For this review, take the finished solid that the model builds, in its own axes (mm). Face numbers are marked on the shaded views. A direction names the side the tool comes from. Round coordinates to 2 decimals unless told otherwise and drop trailing zeros. Write each loop counter-clockwise with the first axis right and the second up, starting at its lowest first coordinate (ties: lowest second). Pieces come first, ordered by that corner, then holes. Notation, with made-up numbers: (35, 7) -> (81, 7) arc R19 ccw to (81, 22) -> close; hole circle Ø11 at (23.5, 53.25). An arc over 180 degrees is marked (long way). Answer in a Markdown table with one row per item.
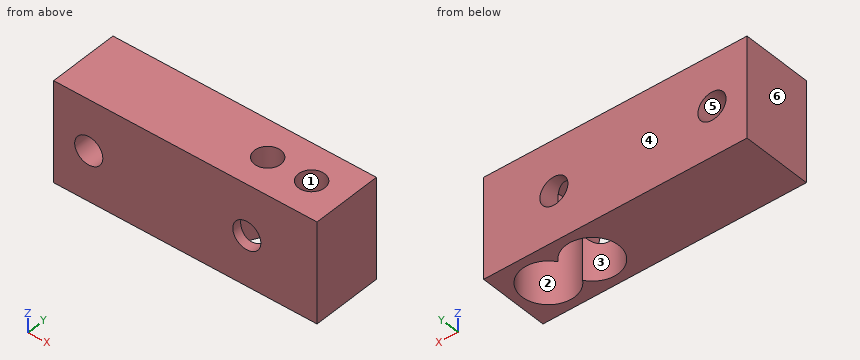
from build123d import *

# Parameters (mm, degrees)
SKETCH1_W           = 30
SKETCH1_H           = 11.5
BOSS_EXTRUDE1_DEPTH = 8
SKETCH2_R           = 1.5
CUT_EXTRUDE1_DEPTH  = 12.5
SKETCH3_R           = 1.598160281
SKETCH3_R_2         = 1.600993429
CUT_EXTRUDE2_DEPTH  = 10
CUT_EXTRUDE3_DEPTH  = 9


with BuildPart() as part:
    # Sketch1 → Boss-Extrude1 (new body)
    with BuildSketch(Plane(origin=(0, 0, 0), x_dir=(1, 0, 0), z_dir=(0, 1, 0))):
        with Locations((15, 5.75)):
            Rectangle(SKETCH1_W, SKETCH1_H)
    extrude(amount=BOSS_EXTRUDE1_DEPTH)

    # Sketch2 → Cut-Extrude1 (cut, through all)
    with BuildSketch(Plane(origin=(0, 0, -11.5), x_dir=(-1, 0, 0), z_dir=(0, 0, -1))):
        with Locations((-21, 4)):
            Circle(SKETCH2_R)
        with Locations((-26, 4)):
            Circle(SKETCH2_R)
    extrude(amount=-CUT_EXTRUDE1_DEPTH, mode=Mode.SUBTRACT)

    # Sketch3 → Cut-Extrude2 (cut)
    with BuildSketch(Plane.XZ):
        with Locations((21.998596175, -5.784390941)):
            Circle(SKETCH3_R)
        with Locations((4.000477604, -5.782705683)):
            Circle(SKETCH3_R_2)
    extrude(amount=-CUT_EXTRUDE2_DEPTH, mode=Mode.SUBTRACT)

    # Sketch4 → Cut-Extrude3 (cut)
    with BuildSketch(Plane(origin=(0, 0, -11.5), x_dir=(-1, 0, 0), z_dir=(0, 0, -1))):
        with BuildLine():
            ThreePointArc((-23.5, 5.658312395), (-29, 4), (-23.5, 2.341687605))
            ThreePointArc((-23.5, 2.341687605), (-18, 4), (-23.5, 5.658312395))
        make_face()
    extrude(amount=-CUT_EXTRUDE3_DEPTH, mode=Mode.SUBTRACT)


solid = part.part
1) Consider section C-C on z = -1.25. State the section outline as (x, y) points.
Solved:
| item | result |
|---|---|
| outline | (0, 0) -> (30, 0) -> (30, 8) -> (0, 8) -> close; hole circle Ø3 at (21, 4); hole circle Ø3 at (26, 4) |
2) Consider section B-B on x = 26. State the section outline as (y, z) points.
Solved:
| item | result |
|---|---|
| outline | (0, -11.5) -> (1, -11.5) -> (1, -2.5) -> (2.5, -2.5) -> (2.5, 0) -> (0, 0) -> close; (5.5, -2.5) -> (7, -2.5) -> (7, -11.5) -> (8, -11.5) -> (8, 0) -> (5.5, 0) -> close |
3) Clearance check with flat-ended pins moving along their axes: pin 1 Ø2.5 at (x, z) = (22, -5.78) entering from -Y; pin 2 Ø3.5 at (x, y) = (21, 4) entering from -Z. State where each tip first meets the part, or that it passes through.
Solved:
| item | result |
|---|---|
| pin 1 | through |
| pin 2 | z = -2.5 |
4) For line 1 (X direction, y = 4, z = -7.75); line 2 (X direction, y = 5.25, z = -5.75); line 3 (X direction, y = 2, z = -4), list the stretches that pass through material, from the lowest coordinate up. Write a range as [from, to].
Solved:
| item | result |
|---|---|
| line 1 | [0, 18], [29, 30] |
| line 2 | [0, 2.4], [5.6, 18.27], [28.73, 30] |
| line 3 | [0, 18.76], [23.24, 23.76], [28.24, 30] |
5) Consider section D-D on y = 1.75. State the section outline as (x, z) points, then the cut area to 3 significant figures.
Solved:
| item | result |
|---|---|
| outline | (0, -11.5) -> (19.02, -11.5) -> (19.02, -2.5) -> (22.98, -2.5) -> (22.98, -4.53) arc R1.6 cw to (22.98, -7.04) -> (22.98, -11.5) -> (24.02, -11.5) -> (24.02, -2.5) -> (27.98, -2.5) -> (27.98, -11.5) -> (30, -11.5) -> (30, 0) -> (0, 0) -> close; hole circle Ø3.2 at (4, -5.78) |
| area | 264 mm² |
6) For the marked faces 1 and 2, list the 3-axis set-ups (+Z, -Z, +X, -X, +Y, -Y) from which the entire face can be reached by the end or side of a thin tool; tool diameter is ignored.
Solved:
| item | result |
|---|---|
| face 1 | +Z, -Z |
| face 2 | -Z |
7) Mouldability with a two-part tool opening along X and no side actions: class the marked faces 3, 4, 5 and 6 as pulls with the +X half, pulls with the -X half, needs draft (parallel to the pull), parting line crosses it, or undercut.
Solved:
| item | result |
|---|---|
| face 3 | undercut |
| face 4 | needs draft |
| face 5 | undercut |
| face 6 | pulls with the -X half |
8) Consider section A-A on y = 4. State the section outline as (x, z) points, then the cut area to 3 significant figures.
Solved:
| item | result |
|---|---|
| outline | (0, -11.5) -> (18, -11.5) -> (18, -2.5) -> (19.5, -2.5) -> (19.5, 0) -> (0, 0) -> close; (22.5, -2.5) -> (24.5, -2.5) -> (24.5, 0) -> (22.5, 0) -> close; (27.5, -2.5) -> (29, -2.5) -> (29, -11.5) -> (30, -11.5) -> (30, 0) -> (27.5, 0) -> close; hole circle Ø3.2 at (4, -5.78) |
| area | 223 mm² |
